Geometry: final body of the model. Coordinates: model frame, mm. Coordinates: 2 decimals unless noted, no trailing zeros. Write each loop counter-clockwise with the first axis right and the second up, starting at its lowest first coordinate (ties: lowest second). Pieces come first, ordered by that corner, then holes. Notation, with made-up numbers: M 74,-2.5 L 87,-2.5 A21 ccw 87,5.5 Z; hole C 3.5,-4 d2. An arc over 180 degrees is marked long. Write item = value, one per line. Start each with the question number.
Item 1: Section D-D on z = 3. Output: boundary loops of the cut face in (x, y).
Item 2: Section C-C on z = 21. Output: boundary loops of the cut face in (x, y), plus the area to 3 significant figures.
Item 3: Section A-A on x = 3.5. Output: boundary loops of the cut face in (y, z).
Item 4: Section B-B on z = 11. Output: boundary loops of the cut face in (x, y), plus the area to 3 significant figures.
Item 5: First-contact query: pin 1 Ø0.5 at (x, y) = (13.5, 1) entering from -Z. Flat tip, straight axial feed; report the tip coordinate or a pass-through.
Item 6: Ray query, L1, parallel to Z at x = 3.5, y = 0.55; L2, parallel to X at y = 0.5, z = 21; L3, parallel to X at y = 0.55, z = 3. Return the intervals inside material, ascending. Write a range as [from, to].
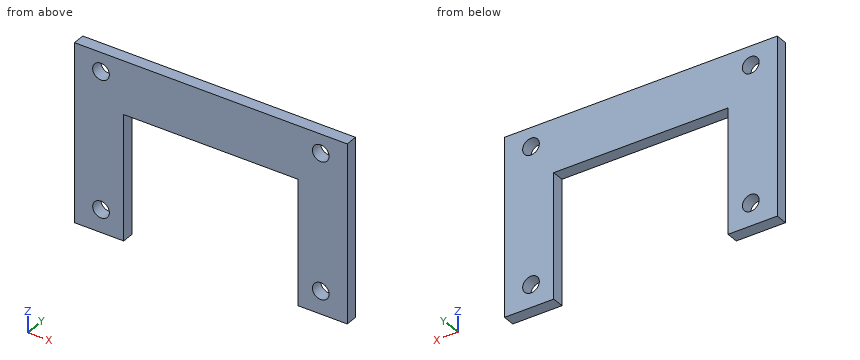
from build123d import *

# Parameters (mm, degrees)
SKETCH_1_W          = 36
SKETCH_1_H          = 24
EXTRUDE_3_DEPTH     = 1.6
SKETCH_3_W          = 22
SKETCH_3_H          = 16
CUT_EXTRUDE_1_DEPTH = 1.6
SKETCH_4_R          = 1.1
CUT_EXTRUDE_2_DEPTH = 1.6
CUT_EXTRUDE_3_DEPTH = 3
SKETCH_6_W          = 36
SKETCH_6_H          = 0.5
CUT_EXTRUDE_4_DEPTH = 3


with BuildPart() as part:
    # 草图1 → 凸台-拉伸3 (new body)
    with BuildSketch(Plane(origin=(0, 0, 0), x_dir=(1, 0, 0), z_dir=(0, 1, 0))):
        with Locations((18, -12)):
            Rectangle(SKETCH_1_W, SKETCH_1_H)
    extrude(amount=EXTRUDE_3_DEPTH)

    # 草图3 → 切除-拉伸1 (cut)
    with BuildSketch(Plane(origin=(0, 1.6, 0), x_dir=(1, 0, 0), z_dir=(0, 1, 0))):
        with Locations((18, -8)):
            Rectangle(SKETCH_3_W, SKETCH_3_H)
    extrude(amount=-CUT_EXTRUDE_1_DEPTH, mode=Mode.SUBTRACT)

    # 草图4 → 切除-拉伸2 (cut)
    with BuildSketch(Plane(origin=(0, 1.6, 0), x_dir=(1, 0, 0), z_dir=(0, 1, 0))):
        with Locations((3.5, -3)):
            Circle(SKETCH_4_R)
        with Locations((32.5, -3)):
            Circle(SKETCH_4_R)
        with Locations((3.5, -21)):
            Circle(SKETCH_4_R)
        with Locations((32.5, -21)):
            Circle(SKETCH_4_R)
    extrude(amount=-CUT_EXTRUDE_2_DEPTH, mode=Mode.SUBTRACT)

    # 草图5 → 切除-拉伸3 (cut)
    with BuildSketch(Plane(origin=(0, 1.6, 0), x_dir=(1, 0, 0), z_dir=(0, 1, 0))):
        Polygon((7, 0), (6.5, 0), (6.5, -16.5), (29.5, -16.5), (29.5, 0), (29, 0), (29, -16), (7, -16), align=None)
    extrude(amount=-CUT_EXTRUDE_3_DEPTH, mode=Mode.SUBTRACT)

    # 草图6 → 切除-拉伸4 (cut)
    with BuildSketch(Plane(origin=(0, 1.6, 0), x_dir=(1, 0, 0), z_dir=(0, 1, 0))):
        with Locations((18, -23.75)):
            Rectangle(SKETCH_6_W, SKETCH_6_H)
    extrude(amount=-CUT_EXTRUDE_4_DEPTH, mode=Mode.SUBTRACT)


solid = part.part
Responses:
q1.outline = M 0,0 L 2.4,0 L 2.4,1.6 L 0,1.6 Z; M 4.6,0 L 6.5,0 L 6.5,1.6 L 4.6,1.6 Z; M 29.5,0 L 31.4,0 L 31.4,1.6 L 29.5,1.6 Z; M 33.6,0 L 36,0 L 36,1.6 L 33.6,1.6 Z
q2.outline = M 0,0 L 2.4,0 L 2.4,1.6 L 0,1.6 Z; M 4.6,0 L 31.4,0 L 31.4,1.6 L 4.6,1.6 Z; M 33.6,0 L 36,0 L 36,1.6 L 33.6,1.6 Z
q2.area = 50.6 mm²
q3.outline = M 0,0 L 1.6,0 L 1.6,1.9 L 0,1.9 Z; M 0,4.1 L 1.6,4.1 L 1.6,19.9 L 0,19.9 Z; M 0,22.1 L 1.6,22.1 L 1.6,23.5 L 0,23.5 Z
q4.outline = M 0,0 L 6.5,0 L 6.5,1.6 L 0,1.6 Z; M 29.5,0 L 36,0 L 36,1.6 L 29.5,1.6 Z
q4.area = 20.8 mm²
q5.pin_1 = 16.5
q6.L1 = [0, 1.9], [4.1, 19.9], [22.1, 23.5]
q6.L2 = [0, 2.4], [4.6, 31.4], [33.6, 36]
q6.L3 = [0, 2.4], [4.6, 6.5], [29.5, 31.4], [33.6, 36]
